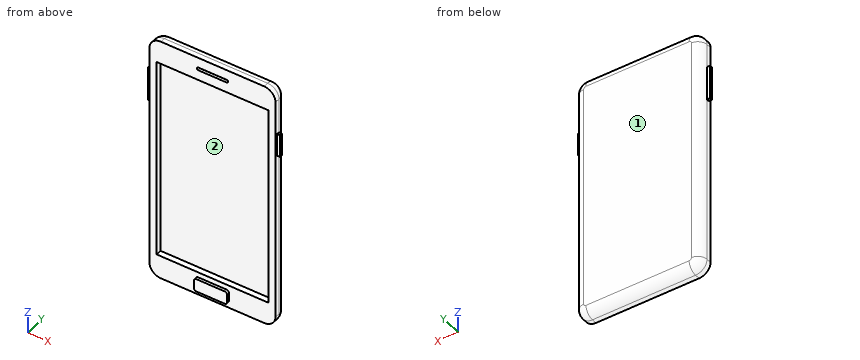
from build123d import *

# Parameters (mm, degrees)
F1_DEPTH  = 7.874
F2_R      = 5.08
F3_W      = 61.9125
F3_H      = 111.125
F4_DEPTH  = 3.175
F6_DEPTH  = 1.5875
F7_DEPTH  = 1.5875
F9_DEPTH  = 1.5875
F11_DEPTH = 1.5875


# Not quite as in the source:
# - a length typed as a fraction of an inch, garbled in the dataset ("3 / 203.2 mm" for 3/8 in), is restored
# - a feature names something its author has since deleted; it is built from what else it names


with BuildPart() as f1:
    # F0 (on Front) → F1 (new body)
    with BuildSketch(Plane.XZ):
        with BuildLine():
            ThreePointArc((-28.575, 68.326), (-33.0651280605, 66.4661280605), (-34.925, 61.976))
            Line((-34.925, 61.976), (-34.925, -61.976))
            ThreePointArc((-34.925, -61.976), (-33.0651280605, -66.4661280605), (-28.575, -68.326))
            Line((-28.575, -68.326), (28.575, -68.326))
            ThreePointArc((28.575, -68.326), (33.0651280605, -66.4661280605), (34.925, -61.976))
            Line((34.925, -61.976), (34.925, 61.976))
            ThreePointArc((34.925, 61.976), (33.0651280605, 66.4661280605), (28.575, 68.326))
            Line((28.575, 68.326), (-28.575, 68.326))
        make_face()
    extrude(amount=F1_DEPTH)

    # F2
    f2_edges = [f1.edges().sort_by_distance(p)[0] for p in [
        (33.065128, 0, 66.466128),
        (0, 0, 68.326),
        (34.925, 0, 0),
    ]]
    fillet(f2_edges, radius=F2_R)

    # F3 (on face) → F4 (cut)
    with BuildSketch(Plane.XZ.offset(7.874)):
        Rectangle(F3_W, F3_H)
    extrude(amount=-F4_DEPTH, mode=Mode.SUBTRACT)

    # F5 (on face) → F6 (join)
    with BuildSketch(Plane.XZ.offset(7.874)):
        with BuildLine():
            Line((7.9375, -58.4327856867), (-7.9375, -58.4327856867))
            ThreePointArc((-7.9375, -58.4327856867), (-8.7591312506, -58.7731164939), (-9.0994620578, -59.5947477445))
            Line((-9.0994620578, -59.5947477445), (-9.0994620578, -64.3572522555))
            ThreePointArc((-9.0994620578, -64.3572522555), (-8.7591311338, -65.1788836228), (-7.9374996698, -65.5192143133))
            Line((-7.9374996698, -65.5192143133), (7.9375003302, -65.5192098023))
            ThreePointArc((7.9375003302, -65.5192098023), (8.7591313673, -65.1788788783), (9.0994620578, -64.3572477445))
            Line((9.0994620578, -64.3572477445), (9.0994620578, -59.5947477445))
            ThreePointArc((9.0994620578, -59.5947477445), (8.7591312506, -58.7731164939), (7.9375, -58.4327856867))
        make_face()
    extrude(amount=F6_DEPTH)

    # F3 (on face) → F7 (cut)
    with BuildSketch(Plane.XZ.offset(7.874)):
        with BuildLine():
            Line((7.9375, 62.76975), (-7.9375, 62.76975))
            ThreePointArc((-7.9375, 62.76975), (-8.4134535744, 62.5726035744), (-8.6106, 62.09665))
            Line((-8.6106, 62.09665), (-8.6106, 61.85535))
            ThreePointArc((-8.6106, 61.85535), (-8.4134535744, 61.3793964256), (-7.9375, 61.18225))
            Line((-7.9375, 61.18225), (7.9375, 61.18225))
            ThreePointArc((7.9375, 61.18225), (8.4134535744, 61.3793964256), (8.6106, 61.85535))
            Line((8.6106, 61.85535), (8.6106, 62.09665))
            ThreePointArc((8.6106, 62.09665), (8.4134535744, 62.5726035744), (7.9375, 62.76975))
        make_face()
    extrude(amount=-F7_DEPTH, mode=Mode.SUBTRACT)

    # F8 (on face) → F9 (join)
    with BuildSketch(Plane(origin=(-34.925, 0, 0), x_dir=(0, -1, 0), z_dir=(-1, 0, 0))):
        with BuildLine():
            Line((6.6675, 30.4519287544), (6.6675, 49.0500712456))
            ThreePointArc((6.6675, 49.0500712456), (6.601327, 49.209827), (6.4415712456, 49.276))
            Line((6.4415712456, 49.276), (5.3059287544, 49.276))
            ThreePointArc((5.3059287544, 49.276), (5.146173, 49.209827), (5.08, 49.0500712456))
            Line((5.08, 49.0500712456), (5.08, 30.4519287544))
            ThreePointArc((5.08, 30.4519287544), (5.146173, 30.292173), (5.3059287544, 30.226))
            Line((5.3059287544, 30.226), (6.4415712456, 30.226))
            ThreePointArc((6.4415712456, 30.226), (6.601327, 30.292173), (6.6675, 30.4519287544))
        make_face()
    extrude(amount=F9_DEPTH)

    # F10 (on face) → F11 (join)
    with BuildSketch(Plane.YZ.offset(34.925)):
        with BuildLine():
            Line((-5.08, 30.4519287544), (-5.08, 42.7000712456))
            ThreePointArc((-5.08, 42.7000712456), (-5.146173, 42.859827), (-5.3059287544, 42.926))
            Line((-5.3059287544, 42.926), (-6.4415712456, 42.926))
            ThreePointArc((-6.4415712456, 42.926), (-6.601327, 42.859827), (-6.6675, 42.7000712456))
            Line((-6.6675, 42.7000712456), (-6.6675, 30.4519287544))
            ThreePointArc((-6.6675, 30.4519287544), (-6.601327, 30.292173), (-6.4415712456, 30.226))
            Line((-6.4415712456, 30.226), (-5.3059287544, 30.226))
            ThreePointArc((-5.3059287544, 30.226), (-5.146173, 30.292173), (-5.08, 30.4519287544))
        make_face()
    extrude(amount=F11_DEPTH)


solid = f1.part
Geometry: final body of the model. Coordinates: model frame, mm. Face numbers are marked on the shaded views. Round coordinates to 2 decimals unless told otherwise and drop trailing zeros. Order: outer loops, then holes, each group sorted by start corner. A loop starts at its lowest first (then second) coordinate and runs counter-clockwise, first axis right, second up. Notation, with made-up numbers: (15, -17) -> (20, -17) arc R38 cw to (20, 22) -> close; hole circle Ø11 at (-13.75, 19.25). An arc over 180 degrees is marked (long way). Put each result on its own line as item: value. Start each with the question number.
Q1. Section A-A on x = -13. Return the cut outline in (y, z).
Q2. Pull-direction query (Z, two-part tool) for the marked faces 1 and 2; classes: +Z half, -Z half, draft (parallel to the pull), parting line (faces both ways), or undercut.
Q3. Line query: probe 1 along Z at (x, y) = (2, -7.5); probe 2 along X at (y, z) = (-5, 7.5); probe 3 along Z at (x, y) = (-11.5, -7). Output: solid intervals per line, ascending.
Q4. Section C-C on z = 34.5. Return the cut outline in (x, y) (1 decimal), and give its area (3 significant figures).
Q5. Section D-D on z = 57.5. Return the cut outline in (x, y) (3 decimals).
Q6. Section B-B on z = -40. Return the cut outline in (x, y) (3 decimals).
Q7. First-contact query: pin 1 (0.5 mm diameter, centred on x = 0, y = -8.5, fed in from +Z); pin 2 (1.5 mm diameter, centred on x = -11, z = -22.5, fed in from -Y); pin 3 (0.5 mm diameter, centred on x = -36, z = 36.5, fed in from -Y); pin 4 (2 mm diameter, centred on x = 22.5, y = -4, fed in from -Z). Flat tips, straight axial feed; report the tip coordinate or a pass-through.
Ans:
1. outline: (-7.87, -68.33) -> (-5.08, -68.33) arc R5.08 ccw to (0, -63.25) -> (0, 63.25) arc R5.08 ccw to (-5.08, 68.33) -> (-7.87, 68.33) -> (-7.87, 55.56) -> (-4.7, 55.56) -> (-4.7, -55.56) -> (-7.87, -55.56) -> close
2. face 1: draft
2. face 2: undercut
3. probe 1: z = -68.33 to -55.56, 55.56 to 61.18, 62.77 to 68.33
3. probe 2: x = -34.92 to -30.96, 30.96 to 34.92
3. probe 3: z = -68.33 to -55.56, 55.56 to 68.33
4. outline: (-36.5, -6.7) -> (-34.9, -6.7) -> (-34.9, -7.9) -> (-31, -7.9) -> (-31, -4.7) -> (31, -4.7) -> (31, -7.9) -> (34.9, -7.9) -> (34.9, -6.7) -> (36.5, -6.7) -> (36.5, -5.1) -> (34.9, -5.1) arc R5.1 ccw to (29.8, 0) -> (-29.8, 0) arc R5.1 ccw to (-34.9, -5.1) -> (-36.5, -5.1) -> close
4. area: 347 mm2
5. outline: (-34.925, -7.874) -> (34.925, -7.874) -> (34.925, -5.08) arc R5.08 ccw to (29.845, 0) -> (-29.845, 0) arc R5.08 ccw to (-34.925, -5.08) -> close
6. outline: (-34.925, -7.874) -> (-30.956, -7.874) -> (-30.956, -4.699) -> (30.956, -4.699) -> (30.956, -7.874) -> (34.925, -7.874) -> (34.925, -5.08) arc R5.08 ccw to (29.845, 0) -> (-29.845, 0) arc R5.08 ccw to (-34.925, -5.08) -> close
7. pin 1: stops at z = -58.43
7. pin 2: stops at y = -4.7
7. pin 3: stops at y = -6.67
7. pin 4: stops at z = -68.33
